from build123d import *

# Parameters (mm, degrees)
F0_W     = 15
F0_H     = 15
F0_W_2   = 14
F0_H_2   = 14
F1_DEPTH = 2
F2_DEPTH = 6
F3_W     = 7.5
F3_H     = 15
F4_DEPTH = 15
F5_R     = 7.49999
F6_R     = 2.5
F7_DEPTH = 25


# Not quite as in the source:
# - a fillet or chamfer is up to 0.001 mm smaller than in the source, because OpenCascade refuses the exact size


with BuildPart() as f1:
    # F0 (on Top) → F1 (new body)
    with BuildSketch(Plane.XY):
        Rectangle(F0_W, F0_H)
        Rectangle(F0_W_2, F0_H_2, mode=Mode.SUBTRACT)
    extrude(amount=F1_DEPTH)

    # F0 (on Top) → F2 (join)
    with BuildSketch(Plane.XY):
        Rectangle(F0_W_2, F0_H_2)
    extrude(amount=F2_DEPTH)

    # F3 (on face) → F4 (join)
    with BuildSketch(Plane(origin=(0, 0, 0), x_dir=(1, 0, 0), z_dir=(0, 0, -1))):
        with Locations((3.75, 0)):
            Rectangle(F3_W, F3_H)
    extrude(amount=F4_DEPTH)

    # F5 (radius 7.5 in the source; OpenCascade refuses exactly that, so slightly less here)
    f5_edges = [f1.edges().sort_by_distance(p)[0] for p in [
        (3.75, 7.5, -15),
        (3.75, -7.5, -15),
    ]]
    fillet(f5_edges, radius=F5_R)

    # F6 (on face) → F7 (cut)
    with BuildSketch(Plane.YZ.offset(7.5)):
        with Locations((0, -7.5)):
            Circle(F6_R)
    extrude(amount=-F7_DEPTH, mode=Mode.SUBTRACT)


solid = f1.part
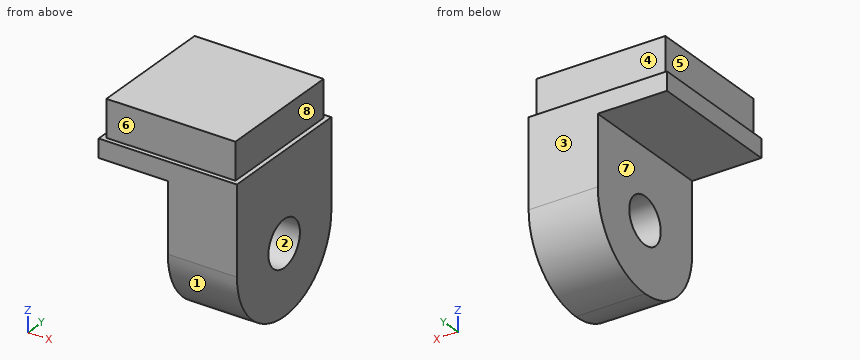
The listing builds one solid part. Answer for the finished solid, in the listing's coordinates (mm). Face numbers are marked on the shaded views. A direction names the side the tool comes from. Give positions to 0.01 mm unless a question says otherwise; leave off trailing zeros. Write each loop counter-clockwise with the first axis right and the second up, starting at its lowest first coordinate (ties: lowest second). Pieces come first, ordered by that corner, then holes.
Item 1: Which of the six approach directions +Z, -Z, +X, -X, +Y, -Y give full straight-line access (tool end or side, diameter ignored) to the marked faces 4, 5, 6, 7 and 8?
Item 2: Section C-C, the plane z = -9.75 is taken. Write down the section's boundary in (x, y), plus the area to 3 significant figures.
Item 3: Determine the mould class of the marked faces 1, 2 and 3 for opening direction Y: released by +Y, released by -Y, zero draft, split by the parting line, or undercut.
Item 4: Section D-D, the plane y = 4.75 is taken. Write down the section's boundary in (x, z).
Item 5: Find the intervals of material crossed by line 1 along Z through (x, y) = (2.5, 0); line 2 along X through (y, z) = (-6.5, -1.75); line 3 along Z through (x, y) = (-6.5, 0), in increasing order.
Item 6: Section B-B, the plane x = -2.5 is taken. Write down the section's boundary in (y, z), plus the area to 3 significant figures.
Item 7: Flat-ended cylindrical pins translate along their axes: P1, Ø3, axis at x = -3, z = 4, coming from the -Y side; P2, Ø8, axis at x = -2, z = -0.5, coming from the +Y side; P3, Ø4.5, axis at x = 1, z = 4.5, coming from the +Y side; P4, Ø3, axis at y = -3, z = 4, coming from the -X side. Find the tip coordinate at first contact, or state that the pin passes through.
Completed:
1. face 4: +Z, +X, -X, +Y
1. face 5: +Z, -X, +Y, -Y
1. face 6: +Z, +X, -X, -Y
1. face 7: -Z, -X, +Y, -Y
1. face 8: +Z, +X, +Y, -Y
2. outline: (0, -7.15) - (7.5, -7.15) - (7.5, -1.09) - (0, -1.09) - close; (0, 1.09) - (7.5, 1.09) - (7.5, 7.15) - (0, 7.15) - close
2. area: 91.0 mm2
3. face 1: released by -Y
3. face 2: undercut
3. face 3: released by +Y
4. outline: (-7.5, 0) - (0, 0) - (0, -13.3) - (7.5, -13.3) - (7.5, 2) - (7, 2) - (7, 6) - (-7, 6) - (-7, 2) - (-7.5, 2) - close
5. line 1: z = -15 to -10, -5 to 6
5. line 2: x = 0 to 7.5
5. line 3: z = 0 to 6
6. outline: (-7.5, 0) - (7.5, 0) - (7.5, 2) - (7, 2) - (7, 6) - (-7, 6) - (-7, 2) - (-7.5, 2) - close
6. area: 86.0 mm2
7. P1: stops at y = -7
7. P2: stops at y = 7.5
7. P3: stops at y = 7
7. P4: stops at x = -7
